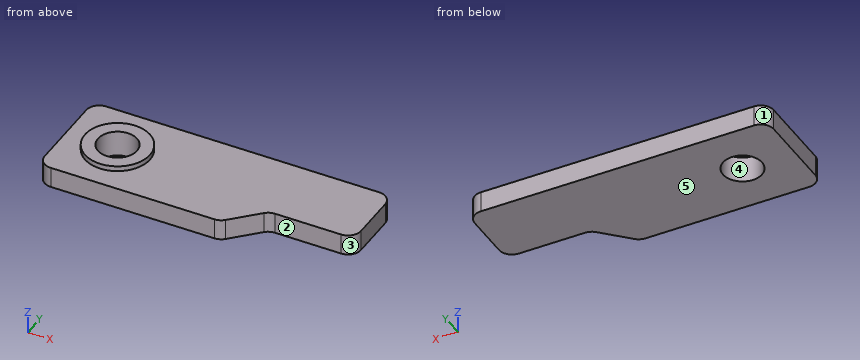
```python
from build123d import *

# Parameters (mm, degrees)
SKETCH1_R           = 1.5
BOSS_EXTRUDE1_DEPTH = 2
SKETCH2_R           = 2.5
CUT_EXTRUDE1_DEPTH  = 0.4
FILLET1_R           = 1


with BuildPart() as part:
    # Sketch1 → Boss-Extrude1 (new body)
    with BuildSketch(Plane.XY):
        Polygon((11.5, -1.5), (5, -1.5), (2.5, -4), (-11.5, -4), (-11.5, 4), (11.5, 4), align=None)
        with Locations((-7.5, 0)):
            Circle(SKETCH1_R, mode=Mode.SUBTRACT)
    extrude(amount=BOSS_EXTRUDE1_DEPTH)

    # Sketch2 → Cut-Extrude1 (cut)
    with BuildSketch(Plane.XY.offset(2)):
        Polygon((-11.5, 4), (-11.5, -4), (2.5, -4), (5, -1.5), (11.5, -1.5), (11.5, 4), align=None)
        with Locations((-7.5, 0)):
            Circle(SKETCH2_R, mode=Mode.SUBTRACT)
    extrude(amount=-CUT_EXTRUDE1_DEPTH, mode=Mode.SUBTRACT)

    # Fillet1
    fillet1_edges = [part.edges().sort_by_distance(p)[0] for p in [
        (-11.5, 4, 0.8),
        (11.5, 4, 0.8),
        (11.5, -1.5, 0.8),
        (5, -1.5, 0.8),
        (2.5, -4, 0.8),
        (-11.5, -4, 0.8),
    ]]
    fillet(fillet1_edges, radius=FILLET1_R)


solid = part.part
```
Part model, mm, in its own coordinate system. Face numbers are marked on the shaded views. A direction names the side the tool comes from. Round coordinates to 2 decimals unless told otherwise and drop trailing zeros. Order: outer loops, then holes, each group sorted by start corner. A loop starts at its lowest first (then second) coordinate and runs counter-clockwise, first axis right, second up. Notation, with made-up numbers: M 54,51 L 67,51 A23 ccw 67,81 Z; hole C 19.25,-12 d11. An arc over 180 degrees is marked long. Put each result on its own line as item: value. Start each with the question number.
1. Slice it at A-A on x = -7.5. List the corners of the cut face in (y, z).
2. Two-plate mould, pull along Y, no slides. Class the marked faces 3, 4 and 5: +Y half, -Y half, draft (parallel to the pull), parting line (faces both ways), or undercut.
3. Slice it at D-D on y = -2. List the corners of the cut face in (x, z), then the cut area to 3 significant figures.
4. Tool access for the marked faces 1 and 2: list every direction of +Z, -Z, +X, -X, +Y, -Y with a clear straight run to the whole face (end or side of a thin tool).
5. Drill centre lines: probe 1 along Y at (x, z) = (-7.5, 0.5); probe 2 along Y at (x, z) = (7.75, 0.25); probe 3 along Z at (x, y) = (5, 0.75). Where is each one in solid material? Low to high. Write a range as [from, to].
6. Slice it at C-C on z = 0.8. List the corners of the cut face in (x, y), then the cut area to 3 significant figures.
7. Drop a flat-ended pin along its axis: pin 1 (0.5 mm diameter, centred on x = 7.5, z = 1, fed in from -Y). Give the stop position or say it passes through.
8. Slice it at B-B on y = 0. List the corners of the cut face in (x, z), then the cut area to 3 significant figures.
Findings:
1. outline: M -4,0 L -1.5,0 L -1.5,2 L -2.5,2 L -2.5,1.6 L -4,1.6 Z; M 1.5,0 L 4,0 L 4,1.6 L 2.5,1.6 L 2.5,2 L 1.5,2 Z
2. face 3: -Y half
2. face 4: undercut
2. face 5: draft
3. outline: M -11.5,0 L 4.5,0 L 4.5,1.6 L -6,1.6 L -6,2 L -9,2 L -9,1.6 L -11.5,1.6 Z
3. area: 26.8 mm2
4. face 1: +Z, -Z, -X, +Y
4. face 2: +Z, -Z, +X, -Y
5. probe 1: [-4, -1.5], [1.5, 4]
5. probe 2: [-1.5, 4]
5. probe 3: [0, 1.6]
6. outline: M -11.5,-3 A1 ccw -10.5,-4 L 2.09,-4 A1 ccw 2.79,-3.71 L 4.71,-1.79 A1 cw 5.41,-1.5 L 10.5,-1.5 A1 ccw 11.5,-0.5 L 11.5,3 A1 ccw 10.5,4 L -10.5,4 A1 ccw -11.5,3 Z; hole C -7.5,0 d3
6. area: 157 mm2
7. pin 1: y = -1.5
8. outline: M -11.5,0 L -9,0 L -9,2 L -10,2 L -10,1.6 L -11.5,1.6 Z; M -6,0 L 11.5,0 L 11.5,1.6 L -5,1.6 L -5,2 L -6,2 Z
8. area: 32.8 mm2
